Source: CAD feature listing. Evaluate the final solid. Frame: model axes, mm. Face numbers are marked on the shaded views. Give positions to 0.01 mm unless a question says otherwise; leave off trailing zeros. Loops run counter-clockwise (first coordinate to the right, second up) from the corner with the lowest first, then second, coordinate; pieces in that order, holes last. Notation, with made-up numbers: M 89,60.25 L 128,60.25 A21 cw 128,92.25 Z; hole C 85,15.25 d4. An arc over 180 degrees is marked long. Answer in a Markdown table with one row per item.
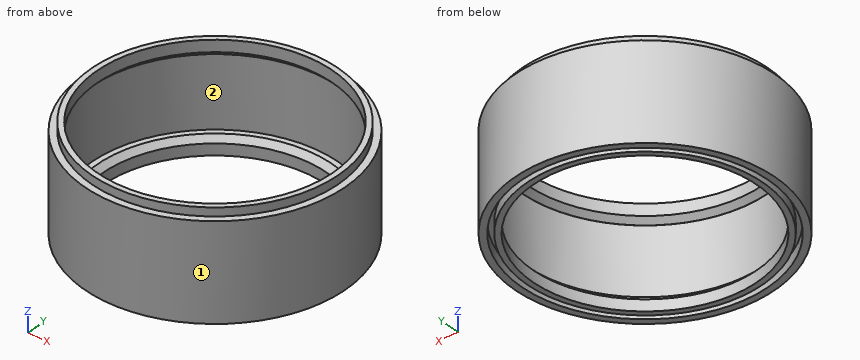
Autodesk Fusion 360 part; units mm, degrees
sketch "chamber" plane through (0, 0, 0) normal (0, 0, 1) x (1, 0, 0)
  circle A0 centre (0, 0) radius 43.825
  circle A1 centre (0, 0) radius 41.875
  circle A2 centre (0, 0) radius 46.25
  circle A3 centre (0, 0) radius 39.85
  dimension "d4" = 87.65
  dimension "d5" = 83.75
  dimension "d6" = 92.5
  dimension "d14" = 79.7
extrude "Extrude1" add sketch "chamber" along normal blind 34 contours A2
extrude "Extrude3" add sketch "chamber" along normal blind 6 from surface at 31 contours A0
extrude "Extrude4" add sketch "chamber" along normal blind 6 contours A0 | A1
extrude "Extrude5" cut sketch "chamber" along normal blind 4 contours A0
chamfer "Chamfer1" distance 2 angle 45 1 edges at (-37.1532, 14.4104, 6)
chamfer "Chamfer2" distance 1.9 angle 45 1 edges at (-39.0412, 15.1426, 31)
equation "ChamberSize = 92.5 mm"
equation "ChamberOffset = 4.8 mm"
equation "ChamberInner = 4 mm"
equation "d4 = ChamberSize - ChamberOffset - 0.05 mm"
equation "d5 = ChamberSize - ChamberOffset - ChamberInner + 0.05 mm"
equation "d6 = ChamberSize"
equation "ChamberHeight = 34 mm"
equation "d8 = ChamberHeight"
equation "ChamberLip = 4 mm"
equation "d14 = ChamberSize - ChamberOffset - ChamberInner - 4 mm"
equation "d15 = ChamberLip + 2 mm"
equation "d17 = ChamberHeight - 3 mm"
Q1. Ray query, probe 1 along Y at (x, z) = (0, 2) (3 decimals); probe 2 along Y at (x, z) = (0, 35) (3 decimals); probe 3 along Y at (x, z) = (0.5, 8). Return the intervals inside material, ascending. Write a range as from..to.
Values follow:
| item | result |
|---|---|
| probe 1 | -46.25..-43.825, -41.875..-39.85, 39.85..41.875, 43.825..46.25 |
| probe 2 | -43.825..-41.875, 41.875..43.825 |
| probe 3 | -46.25..-43.82, 43.82..46.25 |
Q2. Section query C-C (z = 29.5). Output: boundary loops of the cut face in (x, y) (3 decimals), plus the area to 3 significant figures.
Values follow:
| item | result |
|---|---|
| outline | C 0,0 d92.5; hole C 0,0 d87.65 |
| area | 686 mm^2 |
Q3. Mould query, pull axis Y, two halves, no side actions, for the marked faces 1 and 2. Classes: +Y half, -Y half, draft (parallel to the pull), parting line (faces both ways), or undercut.
Values follow:
| item | result |
|---|---|
| face 1 | parting line |
| face 2 | undercut |
Q4. Contact query for flat-ended pins moving along their axis: pin 1 Ø1.5 at (y, z) = (-20.5, 5) entering from -X; pin 2 Ø3 at (y, z) = (-20, 25.5) entering from -X; pin 3 Ø12 at (y, z) = (-17.5, 25.5) entering from +X. Output: stop coordinate, or through.
Values follow:
| item | result |
|---|---|
| pin 1 | x = -41.82 |
| pin 2 | x = -42.39 |
| pin 3 | x = 44.8 |
